Geometry check sheet. Reference: the model listing, model coordinates, mm. A direction names the side the tool comes from. Round coordinates to 2 decimals unless told otherwise and drop trailing zeros. Order: outer loops, then holes, each group sorted by start corner. A loop starts at its lowest first (then second) coordinate and runs counter-clockwise, first axis right, second up.
(1) Sectioned sample at D-D (z = -2.75). Record the boundary of the cut face in (x, y), plus the area to 3 significant figures.
(2) Go/stop test with flat-tipped pins: pin 1 (0.8 mm diameter, centred on x = 0, z = -5, fed in from +Y); pin 2 (5 mm diameter, centred on x = 0, z = 0, fed in from -Y); pin 3 (0.5 mm diameter, centred on y = 11.5, z = -4.5, fed in from +X); pin 4 (0.5 mm diameter, centred on y = 10.5, z = 4.5, fed in from -X). Record where each tip stops, or that it passes through.
(3) Sectioned sample at C-C (x = 1.25). Record the boundary of the cut face in (y, z), plus the area to 3 significant figures.
(4) Set-up check for faces 1 (the face through (-4, 6.22, -2.4)), 2 (the face through (-4.8, 0, 0)): record each of +Z, -Z, +X, -X, +Y, -Y from which the full face is reachable in a straight line by a thin tool's end or side.
(5) Material ranges on line 1 along Z through (x, y) = (0, 12.75) (3 decimals); line 2 along Z through (x, y) = (-1.25, 3.5); line 3 along X through (y, z) = (8.5, -3), recorded low to high.
(6) Release check for a two-part mould opening along Z. For faces 3 (the face through (4.7, 0, 0)), 4 (the face through (3.033, 2.474, -2.964)) record: +Z half, -Z half, draft (parallel to the pull), parting line (faces both ways), or undercut.
(7) Sectioned sample at A-A (y = 12.5). Record the boundary of the cut face in (x, z) (3 decimals).
(8) Sectioned sample at B-B (y = 3.5). Record the boundary of the cut face in (x, z) (3 decimals), plus the area to 3 significant figures.
from build123d import *

# Parameters (mm, degrees)
SKETCH1_R           = 5.065
SKETCH1_R_2         = 3.67
BOSS_EXTRUDE1_DEPTH = 14.17
CUT_EXTRUDE1_DEPTH  = 7.95
SKETCH3_R           = 4.160986794
CUT_EXTRUDE2_DEPTH  = 7.59
CUT_EXTRUDE4_DEPTH  = 5.065
CIRPATTERN2_COUNT   = 6


with BuildPart() as part:
    # Sketch1 → Boss-Extrude1 (new body)
    with BuildSketch(Plane(origin=(0, 0, 0), x_dir=(1, 0, 0), z_dir=(0, 1, 0))):
        Circle(SKETCH1_R)
        Circle(SKETCH1_R_2, mode=Mode.SUBTRACT)
    extrude(amount=BOSS_EXTRUDE1_DEPTH)

    # Sketch2 → Cut-Extrude1 (cut)
    with BuildSketch(Plane(origin=(0, 14.17, 0), x_dir=(1, 0, 0), z_dir=(0, 1, 0))):
        with BuildLine():
            Line((-0.85, 4.362972037), (-0.85, 4.993167832))
            ThreePointArc((-0.85, 4.993167832), (0, 5.065), (0.85, 4.993167832))
            Line((0.85, 4.993167832), (0.85, 4.362972037))
            ThreePointArc((0.85, 4.362972037), (0, 4.445), (-0.85, 4.362972037))
        make_face()
        with BuildLine():
            Line((3.35344462, 2.917607612), (3.899210188, 3.232705509))
            ThreePointArc((3.899210188, 3.232705509), (4.38641867, 2.5325), (4.749210188, 1.760462323))
            Line((4.749210188, 1.760462323), (4.20344462, 1.445364426))
            ThreePointArc((4.20344462, 1.445364426), (3.84948292, 2.2225), (3.35344462, 2.917607612))
        make_face()
        with BuildLine():
            Line((4.20344462, -1.445364426), (4.749210188, -1.760462323))
            ThreePointArc((4.749210188, -1.760462323), (4.38641867, -2.5325), (3.899210188, -3.232705509))
            Line((3.899210188, -3.232705509), (3.35344462, -2.917607612))
            ThreePointArc((3.35344462, -2.917607612), (3.84948292, -2.2225), (4.20344462, -1.445364426))
        make_face()
        with BuildLine():
            Line((0.85, -4.362972037), (0.85, -4.993167832))
            ThreePointArc((0.85, -4.993167832), (0, -5.065), (-0.85, -4.993167832))
            Line((-0.85, -4.993167832), (-0.85, -4.362972037))
            ThreePointArc((-0.85, -4.362972037), (0, -4.445), (0.85, -4.362972037))
        make_face()
        with BuildLine():
            Line((-3.35344462, -2.917607612), (-3.899210188, -3.232705509))
            ThreePointArc((-3.899210188, -3.232705509), (-4.38641867, -2.5325), (-4.749210188, -1.760462323))
            Line((-4.749210188, -1.760462323), (-4.20344462, -1.445364426))
            ThreePointArc((-4.20344462, -1.445364426), (-3.84948292, -2.2225), (-3.35344462, -2.917607612))
        make_face()
        with BuildLine():
            Line((-4.20344462, 1.445364426), (-4.749210188, 1.760462323))
            ThreePointArc((-4.749210188, 1.760462323), (-4.38641867, 2.5325), (-3.899210188, 3.232705509))
            Line((-3.899210188, 3.232705509), (-3.35344462, 2.917607612))
            ThreePointArc((-3.35344462, 2.917607612), (-3.84948292, 2.2225), (-4.20344462, 1.445364426))
        make_face()
    extrude(amount=-CUT_EXTRUDE1_DEPTH, mode=Mode.SUBTRACT)

    # Sketch3 → Cut-Extrude2 (cut)
    with BuildSketch(Plane(origin=(0, 14.17, 0), x_dir=(1, 0, 0), z_dir=(0, 1, 0))):
        Circle(SKETCH3_R)
    extrude(amount=-CUT_EXTRUDE2_DEPTH, mode=Mode.SUBTRACT)

    # Sketch5 → Cut-Extrude4 (cut)
    with BuildSketch(Plane.XY):
        Polygon((0, 4.88), (-2.13, 0), (2.13, 0), align=None)
    cut_extrude4 = extrude(amount=-CUT_EXTRUDE4_DEPTH, mode=Mode.SUBTRACT)

    # CirPattern2: Cut-Extrude4 ×6 about axis
    cirpattern2_axis = Axis((0, 0, 0), (0, 1, 0))
    for i in range(1, CIRPATTERN2_COUNT):
        add(cut_extrude4.rotate(cirpattern2_axis, i * 360 / CIRPATTERN2_COUNT), mode=Mode.SUBTRACT)


solid = part.part
Answer below:
1. outline: (-4.25, 4.3) - (-2.43, 2.21) - (-2.43, 6.58) - (-3.12, 6.58) - (-3.12, 14.17) - (-3.49, 14.17) - (-3.49, 6.22) - (-4.25, 6.22) - close; (2.43, 2.21) - (4.25, 4.3) - (4.25, 6.22) - (3.49, 6.22) - (3.49, 14.17) - (3.12, 14.17) - (3.12, 6.58) - (2.43, 6.58) - close
1. area: 17.2 mm2
2. pin 1: stops at y = 6.22
2. pin 2: passes through
2. pin 3: stops at x = 2.76
2. pin 4: stops at x = -2.76
3. outline: (2.02, -4.91) - (14.17, -4.91) - (14.17, -3.97) - (6.58, -3.97) - (6.58, -3.45) - (2.02, -3.45) - close; (2.02, 3.45) - (6.58, 3.45) - (6.58, 3.97) - (14.17, 3.97) - (14.17, 4.91) - (2.02, 4.91) - close
3. area: 27.6 mm2
4. face 1: +Y
4. face 2: +Z, -Z, +X, -X, -Y
5. line 1: z = -4.445 to -4.161, 4.161 to 4.445
5. line 2: z = -4.91 to -3.45, 3.45 to 4.91
5. line 3: x = -3.5 to -2.88, 2.88 to 3.5
6. face 3: draft
6. face 4: undercut
7. outline: (-4.749, -1.76) - (-4.203, -1.445) arc R4.445 ccw to (-3.353, -2.918) - (-3.899, -3.233) arc R5.065 ccw to (-0.85, -4.993) - (-0.85, -4.363) arc R4.445 ccw to (0.85, -4.363) - (0.85, -4.993) arc R5.065 ccw to (3.899, -3.233) - (3.353, -2.918) arc R4.445 ccw to (4.203, -1.445) - (4.749, -1.76) arc R5.065 ccw to (4.749, 1.76) - (4.203, 1.445) arc R4.445 ccw to (3.353, 2.918) - (3.899, 3.233) arc R5.065 ccw to (0.85, 4.993) - (0.85, 4.363) arc R4.445 ccw to (-0.85, 4.363) - (-0.85, 4.993) arc R5.065 ccw to (-3.899, 3.233) - (-3.353, 2.918) arc R4.445 ccw to (-4.203, 1.445) - (-4.749, 1.76) arc R5.065 ccw to start; hole circle Ø8.322 at (0, 0)
8. outline: (-4.656, -1.993) - (-3.436, -1.288) arc R3.67 cw to (-3.436, 1.288) - (-4.656, 1.993) arc R5.065 ccw to start; (-4.054, -3.036) arc R5.065 ccw to (-0.602, -5.029) - (-0.602, -3.62) arc R3.67 cw to (-2.834, -2.332) - close; (-4.054, 3.036) - (-2.834, 2.332) arc R3.67 cw to (-0.602, 3.62) - (-0.602, 5.029) arc R5.065 ccw to start; (0.602, -5.029) arc R5.065 ccw to (4.054, -3.036) - (2.834, -2.332) arc R3.67 cw to (0.602, -3.62) - close; (0.602, 3.62) arc R3.67 cw to (2.834, 2.332) - (4.054, 3.036) arc R5.065 ccw to (0.602, 5.029) - close; (3.436, -1.288) - (4.656, -1.993) arc R5.065 ccw to (4.656, 1.993) - (3.436, 1.288) arc R3.67 cw to start
8. area: 28.2 mm2
